Build history of the part. All positions in model axes, mm. Face numbers are marked on the shaded views. A direction names the side the tool comes from. Round coordinates to 2 decimals unless told otherwise and drop trailing zeros. Loops run counter-clockwise (first coordinate to the right, second up) from the corner with the lowest first, then second, coordinate; pieces in that order, holes last. Notation, with made-up numbers: (49, 14.5) -> (68, 14.5) arc R17 cw to (68, 47.5) -> close; hole circle Ø6 at (-17.5, 69.25). An arc over 180 degrees is marked (long way). Put each result on its own line as item: value. Start each with the question number.
```python
from build123d import *

# Parameters (mm, degrees)
SKETCH1_R           = 32.5
BOSS_EXTRUDE1_DEPTH = 22
SKETCH2_R           = 5
CUT_EXTRUDE1_DEPTH  = 51.955863254
SKETCH3_R           = 3.349250155
CUT_EXTRUDE2_DEPTH  = 18.804913
CIRPATTERN1_START   = 3.195087105
CIRPATTERN1_DEPTH   = 18.804912895


# Read off the part's stored shape, not the designer's step: CirPattern1
with BuildPart() as part:
    # Sketch1 → Boss-Extrude1 (new body)
    with BuildSketch(Plane(origin=(0, 0, 0), x_dir=(1, 0, 0), z_dir=(0, 1, 0))):
        with Locations(Location((0, 0, 0), (0, 0, 270))):
            Circle(SKETCH1_R)
    extrude(amount=BOSS_EXTRUDE1_DEPTH)

    # Sketch2 → Cut-Extrude1 (cut, through all)
    with BuildSketch(Plane(origin=(0, 0, 0), x_dir=(1, 0, 0), z_dir=(0, 1, 0))):
        with Locations(Location((0, 0, 0), (0, 0, 270))):
            Circle(SKETCH2_R)
    extrude(amount=CUT_EXTRUDE1_DEPTH, mode=Mode.SUBTRACT)

    # Sketch3 → Cut-Extrude2 (cut)
    with BuildSketch(Plane(origin=(0, 22, 0), x_dir=(1, 0, 0), z_dir=(0, 1, 0))):
        with Locations((-7.315673523, 0)):
            Circle(SKETCH3_R)
    extrude(amount=-CUT_EXTRUDE2_DEPTH, mode=Mode.SUBTRACT)

    # CirPattern1 outline → CirPattern1 (cut)
    with BuildSketch(Plane(origin=(0, 0, 0), x_dir=(1, 0, 0), z_dir=(0, 1, 0)).offset(CIRPATTERN1_START)):
        with BuildLine():
            ThreePointArc((-1.960007905, 4.599822715), (0, 5), (1.960007905, 4.599822715))
            ThreePointArc((1.960007905, 4.599822715), (0, 10.664923678), (-1.960007905, 4.599822715))
        make_face()
        with BuildLine():
            ThreePointArc((4.599822715, -1.960007905), (10.664923678, 0), (4.599822715, 1.960007905))
            ThreePointArc((4.599822715, 1.960007905), (5, 0), (4.599822715, -1.960007905))
        make_face()
        with BuildLine():
            ThreePointArc((1.960007905, -4.599822715), (0, -5), (-1.960007905, -4.599822715))
            ThreePointArc((-1.960007905, -4.599822715), (0, -10.664923678), (1.960007905, -4.599822715))
        make_face()
    extrude(amount=CIRPATTERN1_DEPTH, mode=Mode.SUBTRACT)


solid = part.part
```
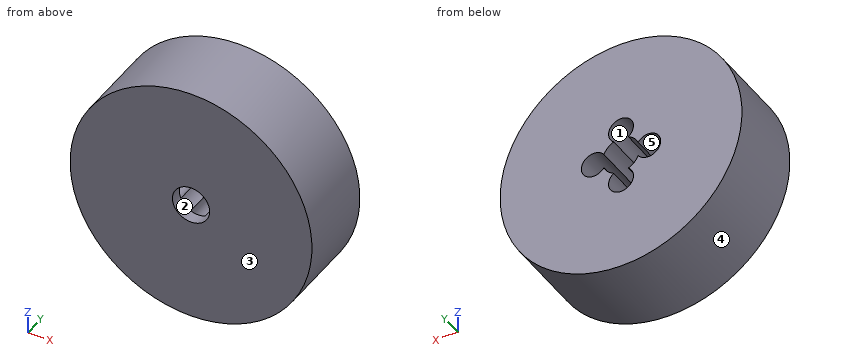
Item 1: Drop flat-ended pins along their axis: pin 1 (1 mm diameter, centred on y = 6.5, z = -14, fed in from -X); pin 2 (6.5 mm diameter, centred on x = -7, z = 1, fed in from +Y); pin 3 (6 mm diameter, centred on x = -7.32, z = 0, fed in from +Y); pin 4 (4 mm diameter, centred on x = -21.5, y = 3.5, fed in from +Z). Give the stop position or say it passes through.
Item 2: Cut at D-D on z = -21.5. Write the cut outline in (x, y).
Item 3: Cut at C-C on x = 0. Write the cut outline in (y, z).
Item 4: Pull direction Z, two halves, no side cores. Call the marked faces 3, 4 and 5: +Z half, -Z half, draft (parallel to the pull), parting line (faces both ways), or undercut.
Item 5: 3-axis set-ups, long thin cutter, end or side, ignore diameter. For the marked faces 1 and 2: which of +Z, -Z, +X, -X, +Y, -Y reach the whole face in a straight line?
Item 6: Cut at A-A on y = 4. Write the cut outline in (x, z).
Item 7: Wall check: line 1 (X direction, y = 16.5, z = 0); line 2 (X direction, y = 17.5, z = 2.5); line 3 (X direction, y = 1.25, z = -2). Give the ranges that are in metal, low to high. Write a range as from..to.
Item 8: Cut at B-B on z = 0. Write the cut outline in (x, y), then the cut area to 3 significant figures.
Ans:
1. pin 1: stops at x = -29.56
1. pin 2: stops at y = 22
1. pin 3: stops at y = 3.2
1. pin 4: stops at z = 26
2. outline: (-24.37, 0) -> (24.37, 0) -> (24.37, 22) -> (-24.37, 22) -> close
3. outline: (0, -32.5) -> (22, -32.5) -> (22, -10.66) -> (3.2, -10.66) -> (3.2, -5) -> (0, -5) -> close; (0, 5) -> (3.2, 5) -> (3.2, 10.66) -> (22, 10.66) -> (22, 32.5) -> (0, 32.5) -> close
4. face 3: draft
4. face 4: parting line
4. face 5: undercut
5. face 1: +Y
5. face 2: +Y, -Y
6. outline: circle Ø65 at (0, 0); hole (-4.6, -1.96) arc R5 ccw to (-1.96, -4.6) arc R3.35 ccw (long way) to (1.96, -4.6) arc R5 ccw to (4.6, -1.96) arc R3.35 ccw (long way) to (4.6, 1.96) arc R5 ccw to (1.96, 4.6) arc R3.35 ccw (long way) to (-1.96, 4.6) arc R5 ccw to (-4.6, 1.96) arc R3.35 ccw (long way) to start
7. line 1: x = -32.5..-10.66, 10.66..32.5
7. line 2: x = -32.4..-9.54, -5.09..-4.33, 4.33..5.09, 9.54..32.4
7. line 3: x = -32.44..-4.58, 4.58..32.44
8. outline: (-32.5, 0) -> (-5, 0) -> (-5, 3.2) -> (-10.66, 3.2) -> (-10.66, 22) -> (-32.5, 22) -> close; (5, 0) -> (32.5, 0) -> (32.5, 22) -> (10.66, 22) -> (10.66, 3.2) -> (5, 3.2) -> close
8. area: 997 mm2
